Autodesk Inventor part; units mm, degrees
ref_plane "YZ Plane" through (0, 0, 0) normal (1, 0, 0) x (0, 1, 0)
ref_plane "XZ Plane" through (0, 0, 0) normal (0, 1, 0) x (-1, 0, 0)
ref_plane "XY Plane" through (0, 0, 0) normal (0, 0, 1) x (1, 0, 0)
sketch "Sketch1" plane through (0, 0, 0) normal (0, 0, 1) x (1, 0, 0)
  line L0 (3.175, 0) -> (41.275, 0)
  line L1 (44.45, 3.175) -> (44.45, 22.225)
  line L2 (41.275, 25.4) -> (3.175, 25.4)
  line L3 (0, 22.225) -> (0, 3.175)
  circle A0 centre (6.35, 12.7) radius 2.0701
  circle A1 centre (31.75, 12.7) radius 2.0701
  arc A2 (3.175, 25.4) -> (0, 22.225) centre (3.175, 22.225) ccw
  arc A3 (44.45, 22.225) -> (41.275, 25.4) centre (41.275, 22.225) ccw
  arc A4 (41.275, 0) -> (44.45, 3.175) centre (41.275, 3.175) ccw
  arc A5 (0, 3.175) -> (3.175, 0) centre (3.175, 3.175) ccw
  circle A6 centre (12.7, 12.7) radius 2.0701
  circle A7 centre (38.1, 12.7) radius 2.0701
  point P0 (0, 0)
  point P1 (44.45, 25.4)
  point P2 (44.45, 0)
  point P3 (0, 25.4)
  dimension "d0" = 44.45
  dimension "d1" = 25.4
  dimension "d2" = 4.1402
  dimension "d3" = 12.7
  dimension "d4" = 6.35
  dimension "d7" = 25.4
  dimension "d21" = 3.175
  dimension "d25" = 4.1402
  dimension "d26" = 12.7
  dimension "d27" = 6.35
  dimension "d30" = 25.4
extrude "Extrusion1" add sketch "Sketch1" along normal blind 6.35
properties part number "Spacer 3" material "Aluminum 6061"
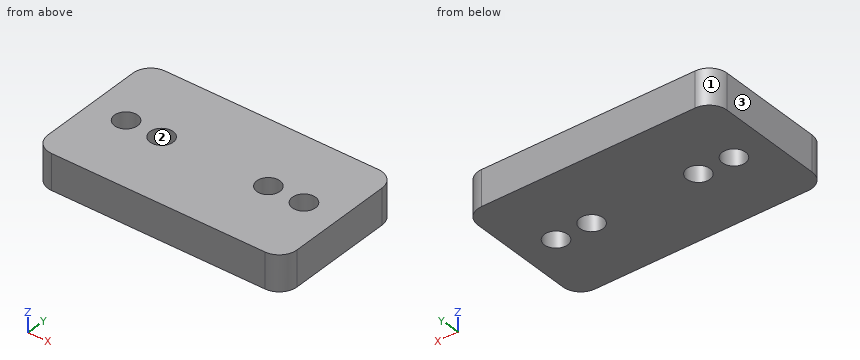
The model under review builds one solid part; all positions refer to its coordinate system, in mm. Face numbers are marked on the shaded views. Coordinates: 2 decimals unless noted, no trailing zeros. Order: outer loops, then holes, each group sorted by start corner. A loop starts at its lowest first (then second) coordinate and runs counter-clockwise, first axis right, second up. Notation, with made-up numbers: (11.25, -35.5) -> (29.25, -35.5) arc R21 ccw to (29.25, -0.5) -> close; hole circle Ø3 at (68, 79). An arc over 180 degrees is marked (long way). Answer in a Markdown table with one row per item.
(1) Consider section B-B (x = 31.75). Write out the cut boundary in (y, z), plus the area to 3 significant figures.
Answers:
| item | result |
|---|---|
| outline | (0, 0) -> (10.63, 0) -> (10.63, 6.35) -> (0, 6.35) -> close; (14.77, 0) -> (25.4, 0) -> (25.4, 6.35) -> (14.77, 6.35) -> close |
| area | 135 mm² |
(2) Consider section A-A (y = 12.7). Write out the cut boundary in (x, z), plus the area to 3 significant figures.
Answers:
| item | result |
|---|---|
| outline | (0, 0) -> (4.28, 0) -> (4.28, 6.35) -> (0, 6.35) -> close; (8.42, 0) -> (10.63, 0) -> (10.63, 6.35) -> (8.42, 6.35) -> close; (14.77, 0) -> (29.68, 0) -> (29.68, 6.35) -> (14.77, 6.35) -> close; (33.82, 0) -> (36.03, 0) -> (36.03, 6.35) -> (33.82, 6.35) -> close; (40.17, 0) -> (44.45, 0) -> (44.45, 6.35) -> (40.17, 6.35) -> close |
| area | 177 mm² |
(3) Consider section C-C (z = 5). Write out the cut boundary in (x, y) (3 decimals).
Answers:
| item | result |
|---|---|
| outline | (0, 3.175) arc R3.175 ccw to (3.175, 0) -> (41.275, 0) arc R3.175 ccw to (44.45, 3.175) -> (44.45, 22.225) arc R3.175 ccw to (41.275, 25.4) -> (3.175, 25.4) arc R3.175 ccw to (0, 22.225) -> close; hole circle Ø4.14 at (6.35, 12.7); hole circle Ø4.14 at (12.7, 12.7); hole circle Ø4.14 at (31.75, 12.7); hole circle Ø4.14 at (38.1, 12.7) |
(4) Insertion check: pin 1 (10 mm diameter, centred on x = 10, y = 22, fed in from -Z); pin 2 (2.5 mm diameter, centred on x = 38.1, y = 12.7, fed in from -Z). Each pin has a flat end and moves straight along its axis. Give the tip position at first contact, or say it passes through.
Answers:
| item | result |
|---|---|
| pin 1 | z = 0 |
| pin 2 | through |
(5) Wall thickness on line 1 along Y through (x, z) = (38.1, 1.5); line 2 along Y through (x, z) = (14.5, 3); line 3 along Y through (x, z) = (42, 2.25): over which ranges is each line inside the solid? List them lowest first.
Answers:
| item | result |
|---|---|
| line 1 | 0 to 10.63, 14.77 to 25.4 |
| line 2 | 0 to 11.68, 13.72 to 25.4 |
| line 3 | 0.08 to 25.32 |
(6) The part is to be moulded in two halves that separate along Y. For the marked faces 1, 2 and 3, say which applies: +Y half, -Y half, draft (parallel to the pull), parting line (faces both ways), or undercut.
Answers:
| item | result |
|---|---|
| face 1 | +Y half |
| face 2 | undercut |
| face 3 | draft |
